Read the model definition and answer for the solid it produces. Units are mm, in the model's axes. A direction names the side the tool comes from. Coordinates: 2 decimals unless noted, no trailing zeros. Write each loop counter-clockwise with the first axis right and the second up, starting at its lowest first coordinate (ties: lowest second). Pieces come first, ordered by that corner, then holes. Notation, with made-up numbers: (66.25, 13.25) -> (96.25, 13.25) arc R26 ccw to (96.25, 47.25) -> close; hole circle Ø6 at (8.25, 6.25). An arc over 180 degrees is marked (long way). Answer in a Markdown table with one row per item. Add a question column.
Item 1: For a pull along X with two mould halves and no side action, classify faces 4 (the face through (0, 0, 0)), 5 (the face through (4.414, -0.108, -0.488)), 6 (the face through (5.65, -0.61, -0.14)) as +X half, -X half, draft (parallel to the pull), parting line (faces both ways), or undercut.
Item 2: Given pin 1 Ø0.6 at (y, z) = (0, 0) entering from -X, flat-ended and moving along its own axis, determine where the tip first touches the part or whether it passes through.
Item 3: Section A-A on x = 7 is taken. Write down the section's boundary in (y, z) (3 decimals), then the cut area to 3 significant figures.
Item 4: Straight lines are drawn through the part: line 1 (Y direction, x = 5.75, z = -0.4); line 2 (Z direction, x = 5, y = 0.3); line 3 (Y direction, x = 7.5, z = -0.4). For each, find the intervals that lie inside material, in ascending order. Write a range as from..to.
Item 5: Which of the six approach directions +Z, -Z, +X, -X, +Y, -Y give full straight-line access (tool end or side, diameter ignored) to faces 1 (the face through (9.6, -0.61, 0.14)), 2 (the face through (11.1, 0, 0)), 3 (the face through (7.649, -0.456, -0.35))?
Item 6: Section B-B on x = 9.75 is taken. Write down the section's boundary in (y, z) (3 decimals).
Autodesk Inventor part; units mm, degrees
ref_plane "Work Plane2" through (3.4, 0, 0) normal (-1, 0, 0) x (0, 0, 1)
ref_plane "Start Plane" through (0, 0, 0) normal (1, 0, 0) x (0, 1, 0)
ref_plane "XZ Plane" through (0, 0, 0) normal (0, 1, 0) x (-1, 0, 0)
sketch "Main Sketch" plane through (0, 0, 0) normal (0, 0, 1) x (1, 0, 0)
  line L0 (0, 0) -> (11.1, 0)
  line L1 (0, 0) -> (0, 0.75)
  line L2 (0, 0.75) -> (0.25, 0.75)
  line L3 (0.25, 0.5) -> (2.082, 0.5)
  line L4 (2.082, 0.575) -> (3.4, 0.575)
  line L5 (3.4, 0.5) -> (5.4, 0.5)
  line L6 (5.4, 0.575) -> (9.85, 0.575)
  line L7 (9.85, 0.5) -> (10.85, 0.5)
  line L8 (11.1, 0.575) -> (11.1, 0)
  line L9 (10.85, 0.575) -> (11.1, 0.575)
  line L10 (0.25, 0.75) -> (0.25, 0.5)
  line L11 (2.082, 0.5) -> (2.082, 0.575)
  line L12 (3.4, 0.575) -> (3.4, 0.5)
  line L13 (5.4, 0.5) -> (5.4, 0.575)
  line L14 (9.85, 0.575) -> (9.85, 0.5)
  line L15 (10.85, 0.5) -> (10.85, 0.575)
  dimension "d3" = 1.5
  dimension "d4" = 1
  dimension "d5" = 1.15
  dimension "d6" = 1
  dimension "d7" = 1.15
  dimension "d8" = 1
  dimension "d9" = 1.15
revolve "Revolution1" add sketch "Main Sketch" angle 360 about axis through (0, 0, 0) along (1, 0, 0)
ref_plane "Work Plane1" through (2.082, 0, 0) normal (-1, 0, 0) x (0, 0, 1)
sketch "Sketch3" plane through (2.082, 0, 0) normal (-1, 0, 0) x (0, 0, 1)
  circle A0 centre (0, 0) radius 0.575
  circle A1 centre (0, 0) radius 0.75
  circle A2 centre (0, 0) radius 0.625
  dimension "d13" = 1.25
extrude "Extrusion1" add sketch "Sketch3" against normal blind 0.5 contours A2
ref_plane "Work Plane2" through (3.4, 0, 0) normal (-1, 0, 0) x (0, 0, 1)
sketch "Sketch4" plane through (3.4, 0, 0) normal (-1, 0, 0) x (0, 0, 1)
  circle A0 centre (0, 0) radius 0.5
  circle A1 centre (0, 0) radius 0.575
  circle A2 centre (0, 0) radius 0.625
  dimension "d17" = 1.25
extrude "Extrusion2" add sketch "Sketch4" along normal blind 0.5 contours A2
sketch "Sketch5" plane through (5.4, 0, 0) normal (-1, 0, 0) x (0, 0, 1)
  circle A0 centre (0, 0) radius 0.575
  circle A1 centre (0, 0) radius 0.625
  dimension "d20" = 1.25
extrude "Extrusion3" add sketch "Sketch5" against normal blind 0.5
sketch "Sketch6" plane through (9.85, 0, 0) normal (1, 0, 0) x (0, 0, -1)
  circle A0 centre (0, 0) radius 0.625
  circle A1 centre (0, 0) radius 0.575
  dimension "d23" = 1.25
extrude "Extrusion4" add sketch "Sketch6" against normal blind 0.5
equation "\"Length\" = 11.1"
properties part number "Shaft" material "Steel"
Results below:
| question | item | result |
|---|---|---|
| 1 | face 4 | -X half |
| 1 | face 5 | undercut |
| 1 | face 6 | draft |
| 2 | pin 1 | stops at x = 0 |
| 3 | outline | circle Ø1.15 at (0, 0) |
| 3 | area | 1.04 mm2 |
| 4 | line 1 | y = -0.48..0.48 |
| 4 | line 2 | z = -0.4..0.4 |
| 4 | line 3 | y = -0.41..0.41 |
| 5 | face 1 | +X |
| 5 | face 2 | +Z, -Z, +X, +Y, -Y |
| 5 | face 3 | none |
| 6 | outline | circle Ø1.25 at (0, 0) |
